Verification items for the finished model (mm, model axes). A direction names the side the tool comes from. Round coordinates to 2 decimals unless told otherwise and drop trailing zeros. Loops run counter-clockwise (first coordinate to the right, second up) from the corner with the lowest first, then second, coordinate; pieces in that order, holes last. Notation, with made-up numbers: M 35,73 L 74,73 A25 ccw 74,85 Z; hole C -25.5,36.25 d4. An arc over 180 degrees is marked long. Answer as CSV lines item,"result".
```python
from build123d import *

# Parameters (mm, degrees)
SKETCH_1_R      = 71
SKETCH_1_R_2    = 68
EXTRUDE_1_DEPTH = 143
EXTRUDE_START   = 54.5
EXTRUDE_8_DEPTH = 25
EXTRUDE_START_2 = 81.5
EXTRUDE_9_DEPTH = 26.5


with BuildPart() as part:
    # 草圖1 → 填料-伸長1 (new body)
    with BuildSketch(Plane(origin=(0, 0, 0), x_dir=(1, 0, 0), z_dir=(0, 1, 0))):
        with Locations(Location((0, 0, 0), (0, 0, 270))):
            Circle(SKETCH_1_R)
        with Locations(Location((0, 0, 0), (0, 0, 270))):
            Circle(SKETCH_1_R_2, mode=Mode.SUBTRACT)
    extrude(amount=EXTRUDE_1_DEPTH)

    # 草圖5 → 填料-伸長8 (add)
    with BuildSketch(Plane(origin=(0, 0, 0), x_dir=(1, 0, 0), z_dir=(0, 1, 0)).offset(EXTRUDE_START)):
        with BuildLine():
            Line((-60.519057708, -31.007154887), (-60.519057708, -11))
            Line((-60.519057708, -11), (-60.519057708, -8.25))
            Line((-60.519057708, -8.25), (-60.519057708, 8.25))
            Line((-60.519057708, 8.25), (-60.519057708, 11))
            Line((-60.519057708, 11), (-60.519057708, 31.007154887))
            ThreePointArc((-60.519057708, 31.007154887), (-68, 0), (-60.519057708, -31.007154887))
        make_face()
        with BuildLine():
            Line((60.519057708, -11), (60.519057708, -31.007154887))
            ThreePointArc((60.519057708, -31.007154887), (66.103312792, -15.948418039), (68, 0))
            ThreePointArc((68, 0), (66.103312792, 15.948418039), (60.519057708, 31.007154887))
            Line((60.519057708, 31.007154887), (60.519057708, 11))
            Line((60.519057708, 11), (60.519057708, 8.25))
            Line((60.519057708, 8.25), (60.519057708, -8.25))
            Line((60.519057708, -8.25), (60.519057708, -11))
        make_face()
    extrude(amount=EXTRUDE_8_DEPTH)

    # 草圖5<10> → 填料-伸長9 (add)
    with BuildSketch(Plane(origin=(0, 0, 0), x_dir=(1, 0, 0), z_dir=(0, 1, 0)).offset(EXTRUDE_START_2)):
        with BuildLine():
            Line((-11, -60.519057708), (-31.007154887, -60.519057708))
            ThreePointArc((-31.007154887, -60.519057708), (0, -68), (31.007154887, -60.519057708))
            Line((31.007154887, -60.519057708), (11, -60.519057708))
            Line((11, -60.519057708), (8.25, -60.519057708))
            Line((8.25, -60.519057708), (-8.25, -60.519057708))
            Line((-8.25, -60.519057708), (-11, -60.519057708))
        make_face()
        with BuildLine():
            ThreePointArc((31.007154887, 60.519057708), (0, 68), (-31.007154887, 60.519057708))
            Line((-31.007154887, 60.519057708), (-11, 60.519057708))
            Line((-11, 60.519057708), (-8.25, 60.519057708))
            Line((-8.25, 60.519057708), (8.25, 60.519057708))
            Line((8.25, 60.519057708), (11, 60.519057708))
            Line((11, 60.519057708), (31.007154887, 60.519057708))
        make_face()
    extrude(amount=EXTRUDE_9_DEPTH)


solid = part.part
```
1) Go/stop test with flat-tipped pins: pin 1 (3 mm diameter, centred on y = 54, z = -53.5, fed in from +X); pin 2 (2 mm diameter, centred on x = 14.5, z = 63.5, fed in from +Y); pin 3 (20 mm diameter, centred on y = 70, z = 13.5, fed in from +X). Record where each tip stops, or that it passes through.
Here are the results:
pin 1,"stops at x = 48.34"
pin 2,"stops at y = 108"
pin 3,"stops at x = 70.91"
2) Set-up check for faces 5 (the flat face through (0, 108, 63)), 6 (the flat face through (0, 95, -60.519)), 7 (the cylindrical face through (2.99, 70.499, -67.934)), 8 (the flat face through (0, 81.5, 63)): record each of +Z, -Z, +X, -X, +Y, -Y from which the full face is reachable in a straight line by a thin tool's end or side.
Here are the results:
face 5,"+Y"
face 6,"+Y, -Y"
face 7,"none"
face 8,"-Y"
3) Section check B-B (x = 0). Record the cut outline in (y, z).
Here are the results:
outline,"M 0,-71 L 143,-71 L 143,-68 L 108,-68 L 108,-60.52 L 81.5,-60.52 L 81.5,-68 L 0,-68 Z; M 0,68 L 81.5,68 L 81.5,60.52 L 108,60.52 L 108,68 L 143,68 L 143,71 L 0,71 Z"
4) Material ranges on probe 1 along X at (y, z) = (98, 0); probe 2 along X at (y, z) = (51, 4); probe 3 along Z at (x, y) = (30.5, 132), recorded low to high.
Here are the results:
probe 1,"x = -71 to -68, 68 to 71"
probe 2,"x = -70.89 to -67.88, 67.88 to 70.89"
probe 3,"z = -64.12 to -60.78, 60.78 to 64.12"
5) Draft check along Z on faces 1 (the cylindrical face through (-62.99, 70.5, 32.76)), 2 (the flat face through (0, 81.5, -63)), 3 (the flat face through (-36, 0, 58)), 4 (the flat face through (63, 79.5, 0)). Enter one of: +Z half, -Z half, draft (parallel to the pull), parting line (faces both ways), or undercut.
Here are the results:
face 1,"parting line"
face 2,"undercut"
face 3,"draft"
face 4,"undercut"
6) Section check C-C (y = 93.5). Record the cut outline in (x, z), plus the area to 3 significant figures.
Here are the results:
outline,"C 0,0 d142; hole M -31.01,-60.52 L 31.01,-60.52 A68 ccw 31.01,60.52 L -31.01,60.52 A68 ccw Z"
area,"1,940 mm^2"
7) Section check D-D (z = -34.5). Record the cut outline in (x, y), plus the area to 3 significant figures.
Here are the results:
outline,"M -62.05,0 L -58.6,0 L -58.6,143 L -62.05,143 Z; M 58.6,0 L 62.05,0 L 62.05,143 L 58.6,143 Z"
area,"988 mm^2"
8) Section check A-A (z = 0). Record the cut outline in (x, y), plus the area to 3 significant figures.
Here are the results:
outline,"M -71,0 L -68,0 L -68,54.5 L -60.52,54.5 L -60.52,79.5 L -68,79.5 L -68,143 L -71,143 Z; M 60.52,54.5 L 68,54.5 L 68,0 L 71,0 L 71,143 L 68,143 L 68,79.5 L 60.52,79.5 Z"
area,"1,230 mm^2"
